Part model, mm, in its own coordinate system. A direction names the side the tool comes from. Give positions to 0.01 mm unless a question says otherwise; leave off trailing zeros. Write each loop counter-clockwise with the first axis right and the second up, starting at its lowest first coordinate (ties: lowest second). Pieces come first, ordered by that corner, then holes.
Autodesk Fusion 360 part; units mm, degrees
sketch "Sketch1" plane through (0, 0, 0) normal (0, 1, 0) x (1, 0, 0)
  circle A0 centre (0, 0) radius 1.75
  dimension "d135" = 3.5
extrude "Extrude1" add sketch "Sketch1" along normal blind 3.5
sketch "Sketch2" plane through (0, 3.5, 0) normal (0, 1, 0) x (-1, 0, 0)
  circle A0 centre (0, 0) radius 1.75
  circle A1 centre (0, 0) radius 3.75
  dimension "d138" = 7.5
extrude "Extrude2" add sketch "Sketch2" along normal blind 2.8 contours A0 | A1
sketch "Sketch3" plane through (0, 0, 0) normal (0, -1, 0) x (1, 0, 0)
  circle A0 centre (0, 0) radius 1.75
  line L0 (1.25, -0.375) -> (-1.25, -0.375)
  line L1 (-1.25, -0.375) -> (-1.25, 0.375)
  line L2 (-1.25, 0.375) -> (1.25, 0.375)
  line L3 (1.25, 0.375) -> (1.25, -0.375)
  line L4 (1.25, -0.375) -> (-1.25, 0.375) construction
  line L5 (-1.25, -0.375) -> (1.25, 0.375) construction
  dimension "d141" = 2.5
  dimension "d142" = 0.75
extrude "Extrude3" cut sketch "Sketch3" against normal blind 2 contours L0 L1 L2 L3
fillet "Fillet1" radius 0.2 4 edges at (-1.25, 0, 0) (0, 0, 0.375) (1.25, 0, 0) (0, 0, -0.375)
fillet "Fillet2" radius 0.1 1 edges at (-1.6316, 0, 0.6328)
fillet "Fillet3" radius 0.2 1 edges at (-1.6316, 3.5, 0.6328)
fillet "Fillet4" radius 0.2 1 edges at (3.4962, 3.5, -1.3561)
chamfer "Chamfer1" distance 0.2 angle 45 1 edges at (3.4962, 6.3, -1.3561)
equation "d135 = Shaft_Dia"
equation "d136 = Shaft_Length"
equation "d138 = Head_Dia"
equation "d139 = Head_Thk"
equation "d141 = Slot_Length"
equation "d142 = Slot_Width"
equation "Head_Dia = 7.5 mm"
equation "Shaft_Dia = 3.5 mm"
equation "Head_Thk = 2.8 mm"
equation "Shaft_Length = 3.5 mm"
equation "Slot_Depth = 2 mm"
equation "Slot_Width = 0.75 mm"
equation "Slot_Length = 2.5 mm"
1) Mould opens along X. For faces 1 (the flat face through (0, 0, 1)), 2 (the cylindrical face through (3.746, 4.883, -0.165)), 3 (the flat face through (0, 1, 0.375)) say: +X half, -X half, draft (parallel to the pull), parting line (faces both ways), or undercut.
Check result:
face 1: draft
face 2: parting line
face 3: undercut
2) Drill centre lines: L1, parallel to X at y = 0.5, z = 0; L2, parallel to Y at x = -1, z = -2.5; L3, parallel to Z at x = -0.75, y = 5.75. Where is each one in solid material? Low to high.
Check result:
L1: x = -1.75 to -1.25, 1.25 to 1.75
L2: y = 3.5 to 6.3
L3: z = -3.67 to 3.67
3) 3-axis set-ups, long thin cutter, end or side, ignore diameter. For faces 4 (the flat face through (0, 1, -0.375)), 5 (the flat face through (0, 6.3, 0)): which of +Z, -Z, +X, -X, +Y, -Y reach the whole face in a straight line?
Check result:
face 4: -Y
face 5: +Z, -Z, +X, -X, +Y
4) Saw through at A-A (z = 0). Write the cut outline in (x, y).
Check result:
outline: (-3.75, 3.7) arc R0.2 ccw to (-3.55, 3.5) - (-1.95, 3.5) arc R0.2 cw to (-1.75, 3.3) - (-1.75, 0.1) arc R0.1 ccw to (-1.65, 0) - (-1.45, 0) arc R0.2 ccw to (-1.25, 0.2) - (-1.25, 2) - (1.25, 2) - (1.25, 0.2) arc R0.2 ccw to (1.45, 0) - (1.65, 0) arc R0.1 ccw to (1.75, 0.1) - (1.75, 3.3) arc R0.2 cw to (1.95, 3.5) - (3.55, 3.5) arc R0.2 ccw to (3.75, 3.7) - (3.75, 6.1) - (3.55, 6.3) - (-3.55, 6.3) - (-3.75, 6.1) - close
5) Saw through at C-C (x = 0). Write the cut outline in (y, z) (3 decimals).
Check result:
outline: (0, -1.65) arc R0.1 ccw to (0.1, -1.75) - (3.3, -1.75) arc R0.2 cw to (3.5, -1.95) - (3.5, -3.55) arc R0.2 ccw to (3.7, -3.75) - (6.1, -3.75) - (6.3, -3.55) - (6.3, 3.55) - (6.1, 3.75) - (3.7, 3.75) arc R0.2 ccw to (3.5, 3.55) - (3.5, 1.95) arc R0.2 cw to (3.3, 1.75) - (0.1, 1.75) arc R0.1 ccw to (0, 1.65) - (0, 0.575) arc R0.2 ccw to (0.2, 0.375) - (2, 0.375) - (2, -0.375) - (0.2, -0.375) arc R0.2 ccw to (0, -0.575) - close
6) Saw through at D-D (y = 5.5). Write the cut outline in (x, z).
Check result:
outline: circle Ø7.5 at (0, 0)
7) Saw through at B-B (y = 1). Write the cut outline in (x, z) (3 decimals).
Check result:
outline: circle Ø3.5 at (0, 0); hole (-1.25, -0.375) - (1.25, -0.375) - (1.25, 0.375) - (-1.25, 0.375) - close
8) Flat gauge pins, fed straight in: P1, Ø1, axis at x = -1.5, z = 1.5, coming from the -Y side; P2, Ø0.9, axis at x = 0.5, y = 1.5, coming from the +Z side; P3, Ø1, axis at x = -1.5, y = 4.5, coming from the +Z side; P4, Ø1.5, axis at x = -0.5, y = 2, coming from the -Z side. Where does each tip first touch, or does it go through?
Check result:
P1: stops at y = 0
P2: stops at z = 1.75
P3: stops at z = 3.61
P4: stops at z = -1.75
